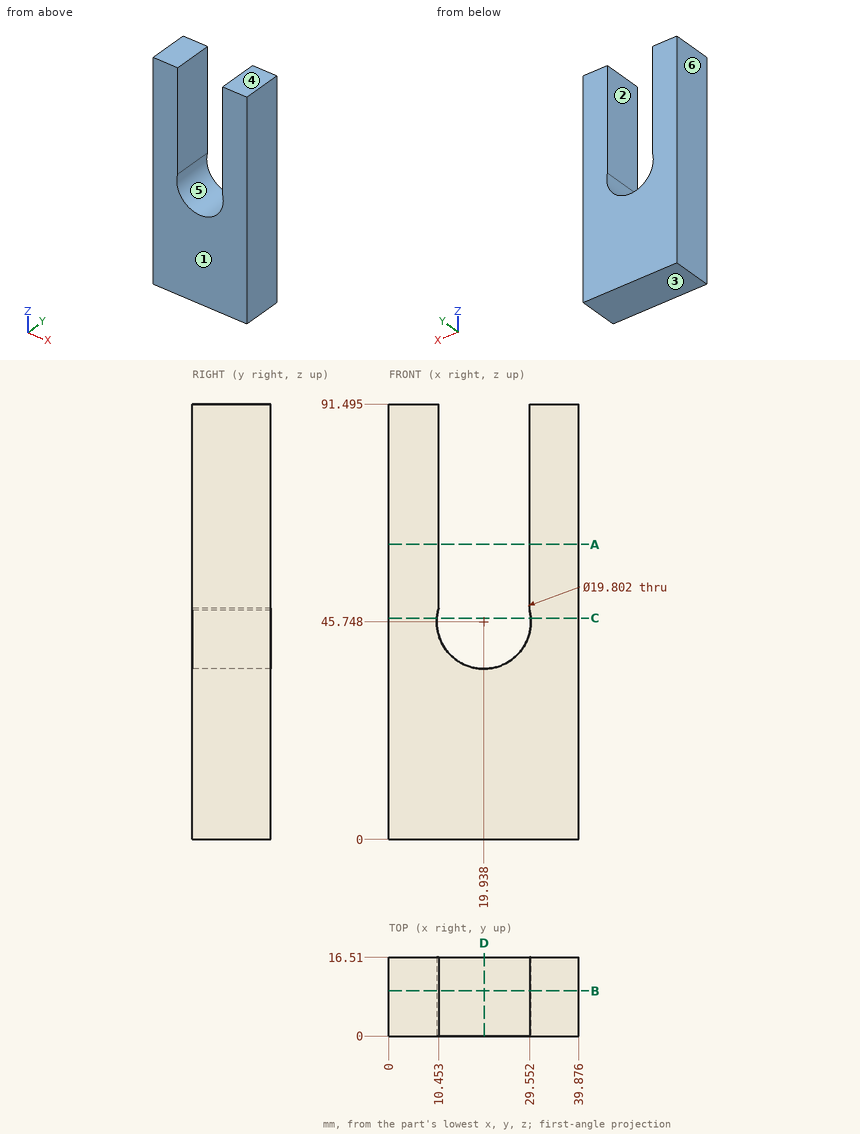
For this review, use the dimensioned drawing (mm, ordinates from the lowest corner) and the shaded views. A direction names the side the tool comes from. Round coordinates to 2 decimals unless told otherwise and drop trailing zeros. Write each loop counter-clockwise with the first axis right and the second up, starting at its lowest first coordinate (ties: lowest second). Pieces come first, ordered by that corner, then holes. Notation, with made-up numbers: (-12.5, -2) -> (-1.5, -2) arc R34 ccw to (-1.5, 29) -> close; hole circle Ø4 at (67.25, -3.75). An arc over 180 degrees is marked (long way). One line per item, written item: value. Start each with the question number.
Q1. Tool access review of the marked faces 1 and 2: name each direction out of +Z, -Z, +X, -X, +Y, -Y from which nothing blocks a thin tool from reaching the whole face with its end or side.
Q2. Add section C-C (z = 46.5). Give the boundary of the cut face in (x, y) (1 decimal), then the cut area to 3 significant figures.
Q3. Add section D-D (x = 20). Give the boundary of the cut face in (y, z), then the cut area to 3 significant figures.
Q4. Add section B-B (y = 9.5). Give the boundary of the cut face in (x, z) (1 decimal).
Q5. Add section A-A (z = 62). Give the boundary of the cut face in (x, y), then the cut area to 3 significant figures.
Q6. To check wall thickness, follow probe 1 along X at (y, z) = (7, 53); probe 2 along X at (y, z) = (6.75, 46.5) (1 decimal); probe 3 along Z at (x, y) = (28, 6.25). State the ranges of each line that lie inside material, in increasing order.
Q7. The part is to be moulded in two halves that separate along Z. For the marked faces 3, 4, 5 and 6, say which applies: pulls with the +Z half, pulls with the -Z half, needs draft (parallel to the pull), parting line crosses it, or undercut.
Response:
1. face 1: +Z, -Z, +X, -X, -Y
1. face 2: +Z, +Y, -Y
2. outline: (0, 0) -> (10.1, 0) -> (10.1, 16.5) -> (0, 16.5) -> close; (29.8, 0) -> (39.9, 0) -> (39.9, 16.5) -> (29.8, 16.5) -> close
2. area: 332 mm^2
3. outline: (0, 0) -> (16.51, 0) -> (16.51, 35.85) -> (0, 35.85) -> close
3. area: 592 mm^2
4. outline: (0, 0) -> (39.9, 0) -> (39.9, 91.5) -> (29.6, 91.5) -> (29.6, 48.1) arc R9.9 cw (long way) to (10.5, 48.6) -> (10.5, 91.5) -> (0, 91.5) -> close
5. outline: (0, 0) -> (10.45, 0) -> (10.45, 16.51) -> (0, 16.51) -> close; (29.55, 0) -> (39.88, 0) -> (39.88, 16.51) -> (29.55, 16.51) -> close
5. area: 343 mm^2
6. probe 1: x = 0 to 10.45, 29.55 to 39.88
6. probe 2: x = 0 to 10.1, 29.8 to 39.9
6. probe 3: z = 0 to 40
7. face 3: pulls with the -Z half
7. face 4: pulls with the +Z half
7. face 5: undercut
7. face 6: needs draft
